Autodesk Inventor part; units mm, degrees
ref_plane "YZ Plane" through (0, 0, 0) normal (1, 0, 0) x (0, 1, 0)
ref_plane "XZ Plane" through (0, 0, 0) normal (0, 1, 0) x (-1, 0, 0)
ref_plane "XY Plane" through (0, 0, 0) normal (0, 0, 1) x (1, 0, 0)
sketch "Sketch44" plane through (0, 0, 0) normal (0, 1, 0) x (-1, 0, 0)
  line L0 (-39.5, 120) -> (39.5, 120)
  line L1 (39.5, 120) -> (39.5, -120)
  line L2 (39.5, -120) -> (-39.5, -120)
  line L3 (-39.5, -120) -> (-39.5, 120)
  line L4 (-39.5, 120) -> (39.5, -120) construction
  line L5 (39.5, 120) -> (-39.5, -120) construction
  point P0 (0, 0)
  dimension "d138" = 79
  dimension "d139" = 240
extrude "Extrusion33" add sketch "Sketch44" along normal blind 3
sketch "Sketch45" plane through (0, 3, 0) normal (0, 1, 0) x (1, 0, 0)
  line L0 (35, -20) -> (-3, -20)
  line L1 (-3, -20) -> (-3, 20)
  line L2 (-3, 20) -> (35, 20)
  line L3 (35, 20) -> (35, -20)
  point P0 (0, 0)
  dimension "d142" = 38
  dimension "d143" = 40
extrude "Extrusion34" add sketch "Sketch45" along normal blind 30
sketch "Sketch47" plane through (0, 0, 0) normal (0, -1, 0) x (1, 0, 0)
  circle A0 centre (16, 0) radius 18
  point P0 (0, 0)
  dimension "d146" = 36
extrude "Extrusion35" cut sketch "Sketch47" against normal blind 30 draft -15
sketch "Sketch58" plane through (35, 3, -20) normal (0, 0, -1) x (-1, 0, 0)
  line L0 (7, 20) -> (27, 20)
  line L1 (27, 20) -> (27, 5)
  line L2 (27, 5) -> (7, 5)
  line L3 (7, 5) -> (7, 20)
  point P0 (35, -3)
  dimension "d156" = 20
  dimension "d157" = 15
extrude "Extrusion38" cut sketch "Sketch58" against normal blind 15
sketch "Sketch59" plane through (-3, 3, -20) normal (-1, 0, 0) x (0, 0, 1)
  line L0 (4.5, 25) -> (8, 25)
  line L1 (8, 25) -> (8, 5)
  line L2 (8, 5) -> (4.5, 5)
  line L3 (4.5, 5) -> (4.5, 25)
  point P0 (20, -3)
  dimension "d160" = 3.5
  dimension "d161" = 20
extrude "Extrusion39" cut sketch "Sketch59" against normal blind 35
sketch "Sketch60" plane through (0, 3, 0) normal (0, 1, 0) x (1, 0, 0)
  line L0 (-33.965, 38.3247) -> (-28.965, 38.3247)
  line L1 (-28.965, 38.3247) -> (-28.965, 58.3247)
  line L2 (-28.965, 58.3247) -> (-33.965, 58.3247)
  line L3 (-33.965, 58.3247) -> (-33.965, 38.3247)
  point P0 (0, 0)
  dimension "d164" = 5
  dimension "d165" = 20
extrude "Extrusion40" add sketch "Sketch60" along normal blind 20
sketch "Sketch61" plane through (0, 23, 0) normal (0, 1, 0) x (1, 0, 0)
  line L0 (-28.965, 38.3247) -> (-28.965, 58.3247)
  line L1 (-28.965, 38.3247) -> (-48.965, 38.3247)
  line L2 (-48.965, 38.3247) -> (-48.965, 58.3247)
  line L3 (-48.965, 58.3247) -> (-28.965, 58.3247)
  line L4 (-28.965, 58.3247) -> (-28.965, 38.3247)
  point P0 (0, 0)
  dimension "d168" = 20
  dimension "d169" = 20
extrude "Extrusion41" add sketch "Sketch61" against normal blind 5
sketch "Sketch65" plane through (-3, 3, -20) normal (-1, 0, 0) x (0, 0, 1)
  circle A0 centre (20, 15) radius 3
  point P0 (20, -3)
  dimension "d176" = 6
extrude "Extrusion43" cut sketch "Sketch65" against normal blind 10
sketch "Sketch68" plane through (0, 3, 0) normal (0, 1, 0) x (1, 0, 0)
  circle A0 centre (-31.5, -112) radius 3.35
  circle A1 centre (31.5, -112) radius 3.35
  circle A2 centre (-31.5, 112) radius 3.35
  circle A3 centre (31.5, 112) radius 3.35
  point P0 (0, 0)
  dimension "d192" = 6.7
  dimension "d193" = 6.7
  dimension "d194" = 6.7
  dimension "d195" = 6.7
extrude "Extrusion46" cut sketch "Sketch68" against normal through all
sketch "Sketch69" plane through (0, 3, 0) normal (0, 1, 0) x (1, 0, 0)
  circle A0 centre (23.5, -27) radius 3.35
  circle A1 centre (23.5, 27) radius 3.35
  point P0 (0, 0)
  dimension "d198" = 6.7
  dimension "d199" = 6.7
extrude "Extrusion47" cut sketch "Sketch69" against normal through all
sketch "Sketch70" plane through (0, 0, 0) normal (0, -1, 0) x (1, 0, 0)
  line L0 (-3, -12) -> (32, -12)
  line L1 (2.479, -12) -> (29.6644, -12)
  line L2 (29.6644, -12) -> (29.6644, -18.105)
  line L3 (29.6644, -18.105) -> (2.479, -18.105)
  line L4 (2.479, -18.105) -> (2.479, -12)
  point P0 (0, 0)
extrude "Extrusion48" add sketch "Sketch70" against normal blind 8
sketch "Sketch71" plane through (0, 33, 0) normal (0, 1, 0) x (1, 0, 0)
  point P0 (0, 0)
sketch "Sketch73" plane through (0, 33, 0) normal (0, 1, 0) x (1, 0, 0)
  circle A0 centre (20, 0) radius 1.1
  point P0 (0, 0)
  dimension "d207" = 2.2
extrude "Extrusion50" cut sketch "Sketch73" against normal blind 10
equation "\"d193\" = d192"
equation "\"d194\" = d192"
equation "\"d195\" = d192"
equation "\"d198\" = d192"
equation "\"d199\" = d192"
properties part number "liquid port_v09"
The model under review builds one solid part; all positions refer to its coordinate system, in mm. A direction names the side the tool comes from. Round coordinates to 2 decimals unless told otherwise and drop trailing zeros. Order: outer loops, then holes, each group sorted by start corner. A loop starts at its lowest first (then second) coordinate and runs counter-clockwise, first axis right, second up. Notation, with made-up numbers: (51, 49) -> (81, 49) arc R22 ccw to (81, 56) -> close; hole circle Ø5 at (81, 17.5). An arc over 180 degrees is marked (long way). Return JSON: item names as keys, results as strings.
1. Take a section at C-C (z = 27). Write out the cut boundary in (x, y), then the cut area to 3 significant figures.
Answer block:
{"outline": "(-39.5, 0) -> (20.15, 0) -> (20.15, 3) -> (-39.5, 3) -> close; (26.85, 0) -> (39.5, 0) -> (39.5, 3) -> (26.85, 3) -> close", "area": "217 mm²"}
2. Take a section at D-D (x = 16). Write out the cut boundary in (y, z), then the cut area to 3 significant figures.
Answer block:
{"outline": "(0, -120) -> (3, -120) -> (3, -20) -> (8, -20) -> (8, -12) -> (0, -12) -> close; (0, 18) -> (30, 9.96) -> (30, -9.96) -> (23, -11.84) -> (23, -12) -> (28, -12) -> (28, -15.5) -> (23, -15.5) -> (23, -20) -> (33, -20) -> (33, 20) -> (3, 20) -> (3, 120) -> (0, 120) -> close", "area": "1,010 mm²"}
3. For faces 4 (the face through (-32, 17, -58.325)), 5 (the face through (28, 17, -9)), 6 (the face through (14, 8, -15)), list the 3-axis set-ups (+Z, -Z, +X, -X, +Y, -Y) from which the entire face can be reached by the end or side of a thin tool; tool diameter is ignored.
Answer block:
{"face 4": "-Z, +X, -X, +Y", "face 5": "-Z", "face 6": "none"}
4. Insertion check: P1, Ø15, axis at x = 14, y = 24.5, coming from the +Z side; P2, Ø6, axis at x = 31.5, z = -112, coming from the -Y side; P3, Ø3.5, axis at x = 20, z = 0, coming from the -Y side; P4, Ø16, axis at y = 18, z = -46, coming from the +X side (3 decimals). Each pin has a flat end and moves straight along its axis. Give the tip position at first contact, or say it passes through.
Answer block:
{"P1": "stops at z = 20", "P2": "passes through", "P3": "stops at y = 30", "P4": "stops at x = -28.965"}
5. For L1, parallel to Z at x = 2.5, y = 18; L2, parallel to X at y = 1.85, z = 27; L3, parallel to Y at x = 14, z = -17, list the stretches that pass through material, from the lowest coordinate up. Write a range as [from, to].
Answer block:
{"L1": "z = [-20, -15.5], [-12, -3], [3, 20]", "L2": "x = [-39.5, 20.15], [26.85, 39.5]", "L3": "y = [0, 8], [23, 33]"}
6. The part is to be moulded in two halves that separate along X. For faces 1 (the face through (-48.965, 21, -48)), 2 (the face through (-28.305, 1.521, -113.006)), 3 (the face through (35, 18, 0)), say which applies: +X half, -X half, draft (parallel to the pull), parting line (faces both ways), or undercut.
Answer block:
{"face 1": "-X half", "face 2": "undercut", "face 3": "+X half"}
7. Take a section at B-B (y = 11). Write out the cut boundary in (x, z) (3 decimals).
Answer block:
{"outline": "(-33.965, -58.325) -> (-28.965, -58.325) -> (-28.965, -38.325) -> (-33.965, -38.325) -> close; (-3, -20) -> (8, -20) -> (8, -15.5) -> (-3, -15.5) -> close; (-3, -12) -> (6.913, -12) arc R15.053 cw (long way) to (28, -9.087) -> (28, -12) -> (32, -12) -> (32, -15.5) -> (28, -15.5) -> (28, -20) -> (35, -20) -> (35, 20) -> (-3, 20) -> close"}
8. Take a section at A-A (z = -112). Write out the cut boundary in (x, y), then the cut area to 3 significant figures.
Answer block:
{"outline": "(-39.5, 0) -> (-34.85, 0) -> (-34.85, 3) -> (-39.5, 3) -> close; (-28.15, 0) -> (28.15, 0) -> (28.15, 3) -> (-28.15, 3) -> close; (34.85, 0) -> (39.5, 0) -> (39.5, 3) -> (34.85, 3) -> close", "area": "197 mm²"}
